```python
from build123d import *

# Parameters (mm, degrees)
SKETCH_1_W                       = 560
SKETCH_1_H                       = 144
EXTRUDE_7_DEPTH                  = 18
SKETCH_2_R                       = 11
CUT_EXTRUDE_2_DEPTH              = 579.498055312
PATTERN_LINEAR_2_COUNT           = 2
PATTERN_LINEAR_2_PITCH           = 80
PATTERN_LINEAR_2_COUNT_DIR2      = 3
PATTERN_LINEAR_2_PITCH_DIR2      = 80
PATTERN_LINEAR_4_COUNT           = 2
PATTERN_LINEAR_4_PITCH           = 320
PATTERN_LINEAR_4_COPY_1_SKETCH_R = 11
PATTERN_LINEAR_4_COPY_1_DEPTH    = 579.498055312
PATTERN_LINEAR_4_COPY_2_SKETCH_R = 11
PATTERN_LINEAR_4_COPY_2_DEPTH    = 579.498055312
PATTERN_LINEAR_4_COPY_3_SKETCH_R = 11
PATTERN_LINEAR_4_COPY_3_DEPTH    = 579.498055312
PATTERN_LINEAR_4_COPY_4_SKETCH_R = 11
PATTERN_LINEAR_4_COPY_4_DEPTH    = 579.498055312
PATTERN_LINEAR_4_COPY_5_SKETCH_R = 11
PATTERN_LINEAR_4_COPY_5_DEPTH    = 579.498055312


with BuildPart() as part:
    # 草图1 → 拉伸7 (new body)
    with BuildSketch(Plane.XY):
        with Locations((280, 72)):
            Rectangle(SKETCH_1_W, SKETCH_1_H)
    extrude(amount=EXTRUDE_7_DEPTH)

    # 草图2 → 切除-拉伸2 (cut, through all)
    with BuildSketch(Plane.XY.offset(18)):
        with Locations((40, 112)):
            Circle(SKETCH_2_R)
    cut_extrude_2 = extrude(amount=-CUT_EXTRUDE_2_DEPTH, mode=Mode.SUBTRACT)

    # 阵列(线性)2: Cut-Extrude 2 2 × 3
    with Locations(*[(j * PATTERN_LINEAR_2_PITCH_DIR2, -i * PATTERN_LINEAR_2_PITCH, 0) for i in range(PATTERN_LINEAR_2_COUNT) for j in range(PATTERN_LINEAR_2_COUNT_DIR2) if (i, j) != (0, 0)]):
        add(cut_extrude_2, mode=Mode.SUBTRACT)

    # 阵列(线性)4: 切除-拉伸2 ×2
    with Locations(*[(i * PATTERN_LINEAR_4_PITCH, 0, 0) for i in range(1, PATTERN_LINEAR_4_COUNT)]):
        add(cut_extrude_2, mode=Mode.SUBTRACT)

    # 阵列(线性)4 copy 1 sketch → 阵列(线性)4 copy 1 (cut, through all)
    with BuildSketch(Plane(origin=(400, 0, 18), x_dir=(1, 0, 0), z_dir=(0, 0, 1))):
        with Locations((40, 112)):
            Circle(PATTERN_LINEAR_4_COPY_1_SKETCH_R)
    extrude(amount=-PATTERN_LINEAR_4_COPY_1_DEPTH, mode=Mode.SUBTRACT)

    # 阵列(线性)4 copy 2 sketch → 阵列(线性)4 copy 2 (cut, through all)
    with BuildSketch(Plane(origin=(480, 0, 18), x_dir=(1, 0, 0), z_dir=(0, 0, 1))):
        with Locations((40, 112)):
            Circle(PATTERN_LINEAR_4_COPY_2_SKETCH_R)
    extrude(amount=-PATTERN_LINEAR_4_COPY_2_DEPTH, mode=Mode.SUBTRACT)

    # 阵列(线性)4 copy 3 sketch → 阵列(线性)4 copy 3 (cut, through all)
    with BuildSketch(Plane(origin=(320, -80, 18), x_dir=(1, 0, 0), z_dir=(0, 0, 1))):
        with Locations((40, 112)):
            Circle(PATTERN_LINEAR_4_COPY_3_SKETCH_R)
    extrude(amount=-PATTERN_LINEAR_4_COPY_3_DEPTH, mode=Mode.SUBTRACT)

    # 阵列(线性)4 copy 4 sketch → 阵列(线性)4 copy 4 (cut, through all)
    with BuildSketch(Plane(origin=(400, -80, 18), x_dir=(1, 0, 0), z_dir=(0, 0, 1))):
        with Locations((40, 112)):
            Circle(PATTERN_LINEAR_4_COPY_4_SKETCH_R)
    extrude(amount=-PATTERN_LINEAR_4_COPY_4_DEPTH, mode=Mode.SUBTRACT)

    # 阵列(线性)4 copy 5 sketch → 阵列(线性)4 copy 5 (cut, through all)
    with BuildSketch(Plane(origin=(480, -80, 18), x_dir=(1, 0, 0), z_dir=(0, 0, 1))):
        with Locations((40, 112)):
            Circle(PATTERN_LINEAR_4_COPY_5_SKETCH_R)
    extrude(amount=-PATTERN_LINEAR_4_COPY_5_DEPTH, mode=Mode.SUBTRACT)


solid = part.part
```
CAD build for the part. Positions are in the model's coordinates, mm. Give positions to 0.01 mm unless a question says otherwise; leave off trailing zeros. Order: outer loops, then holes, each group sorted by start corner. A loop starts at its lowest first (then second) coordinate and runs counter-clockwise, first axis right, second up.
(1) Mould opens along X. For faces 1 (the flat face through (276, 73, 0)), 2 (the cylindrical face through (429, 32, 9)), 3 (the flat face through (560, 71, 9)), 4 (the flat face through (0, 71, 9)) say: released by +X, released by -X, zero draft, split by the parting line, or undercut.
(2) Saw through at D-D, the plane x = 514.5. Give the cut face in (y, z).
(3) Drill centre lines: L1, parallel to Y at x = 360, z = 5.5; L2, parallel to Y at x = 196.5, z = 2.5. Where is each one in solid material? Low to high.
(4) Flat gauge pin, fed straight in: pin 1 (20 mm diameter, centred on x = 520, y = 112, fed in from +Z). Where does the tip first touch, or does it go through?
(5) Saw through at A-A, the plane z = 4. State how many separate pieces and enclosed holes the cut face has, then the cut area to 3 significant figures.
(6) Saw through at C-C, the plane y = 112. Give the cut face in (x, z).
(7) Saw through at B-B, the plane x = 360. Give the cut face in (y, z).
Results found:
1. face 1: zero draft
1. face 2: undercut
1. face 3: released by +X
1. face 4: released by -X
2. outline: (0, 0) - (22.47, 0) - (22.47, 18) - (0, 18) - close; (41.53, 0) - (102.47, 0) - (102.47, 18) - (41.53, 18) - close; (121.53, 0) - (144, 0) - (144, 18) - (121.53, 18) - close
3. L1: y = 0 to 21, 43 to 101, 123 to 144
3. L2: y = 0 to 21.57, 42.43 to 101.57, 122.43 to 144
4. pin 1: passes through
5. separate pieces: 1
5. enclosed holes: 12
5. area: 76,100 mm2
6. outline: (0, 0) - (29, 0) - (29, 18) - (0, 18) - close; (51, 0) - (109, 0) - (109, 18) - (51, 18) - close; (131, 0) - (189, 0) - (189, 18) - (131, 18) - close; (211, 0) - (349, 0) - (349, 18) - (211, 18) - close; (371, 0) - (429, 0) - (429, 18) - (371, 18) - close; (451, 0) - (509, 0) - (509, 18) - (451, 18) - close; (531, 0) - (560, 0) - (560, 18) - (531, 18) - close
7. outline: (0, 0) - (21, 0) - (21, 18) - (0, 18) - close; (43, 0) - (101, 0) - (101, 18) - (43, 18) - close; (123, 0) - (144, 0) - (144, 18) - (123, 18) - close
